Input: part model. Units: mm. Frame: model coordinates. A direction names the side the tool comes from. Round coordinates to 2 decimals unless told otherwise and drop trailing zeros. Loops run counter-clockwise (first coordinate to the right, second up) from the corner with the lowest first, then second, coordinate; pieces in that order, holes last. Notation, with made-up numbers: M 72,83 L 125,83 A9 ccw 125,94 Z; hole C -31.75,66.5 d9. An arc over 180 degrees is marked long. Put each result on its own line as item: value. Start each with the question number.
1) Line query: probe 1 along Y at (x, z) = (-13, 6.5); probe 2 along X at (y, z) = (33, 0.5); probe 3 along Z at (x, y) = (-10, 50). Output: solid intervals per line, ascending.
2) Section D-D on z = 0. Output: boundary loops of the cut face in (x, y).
3) Section A-A on x = 0. Output: boundary loops of the cut face in (y, z).
4) Pin query (flat end, axial travel): pin 1 (10 mm diameter, centred on x = -13, z = 4.5, fed in from -Y); pin 2 (1.5 mm diameter, centred on y = 51.5, z = -1, fed in from +X); pin 3 (5 mm diameter, centred on y = 57, z = 5.5, fed in from -X); pin 4 (12 mm diameter, centred on y = 57, z = -1.5, fed in from -X). Return the tip coordinate at first contact, or that it passes through.
5) Reachability of faces 1 (the face through (0, 77, 5.082)), 2 (the face through (0, 0, 0)) from +Z, -Z, +X, -X, +Y, -Y: full face, straight path, thin tool, end or side. Return the list, or none.
6) Section C-C on y = 16. Output: boundary loops of the cut face in (x, z), plus the area to 3 significant figures.
7) Section B-B on z = 9. Output: boundary loops of the cut face in (x, y), plus the area to 3 significant figures.
from build123d import *

# Parameters (mm, degrees)
SKETCH1_R           = 19.05
BOSS_EXTRUDE1_DEPTH = 76.2
BOSS_EXTRUDE3_DEPTH = 2.54


with BuildPart() as part:
    # Sketch1 → Boss-Extrude1 (new body)
    with BuildSketch(Plane(origin=(0, 0, 0), x_dir=(1, 0, 0), z_dir=(0, 1, 0))):
        with Locations(Location((0, 0, 0), (0, 0, 90))):
            Circle(SKETCH1_R)
    extrude(amount=BOSS_EXTRUDE1_DEPTH)

    # Sketch2 → Boss-Extrude3 (add)
    with BuildSketch(Plane(origin=(0, 76.2, 0), x_dir=(1, 0, 0), z_dir=(0, 1, 0))):
        with BuildLine():
            Line((2.273328114, -5.081659317), (0, -5.081659317))
            Line((0, -5.081659317), (-2.273328114, -5.081659317))
            ThreePointArc((-2.273328114, -5.081659317), (-1.086554166, -9.959754211), (3.048, -7.112))
            ThreePointArc((3.048, -7.112), (2.847754211, -6.025445834), (2.273328114, -5.081659317))
        make_face()
    extrude(amount=BOSS_EXTRUDE3_DEPTH)


solid = part.part
Geometry results:
1. probe 1: y = 0 to 76.2
1. probe 2: x = -19.04 to 19.04
1. probe 3: z = -16.21 to 16.21
2. outline: M -19.05,0 L 19.05,0 L 19.05,76.2 L -19.05,76.2 Z
3. outline: M 0,-19.05 L 76.2,-19.05 L 76.2,5.08 L 78.74,5.08 L 78.74,10.16 L 76.2,10.16 L 76.2,19.05 L 0,19.05 Z
4. pin 1: stops at y = 0
4. pin 2: stops at x = 19.05
4. pin 3: stops at x = -18.81
4. pin 4: stops at x = -19.05
5. face 1: -Z, +X, -X, +Y
5. face 2: +Z, -Z, +X, -X, -Y
6. outline: C 0,0 d38.1
6. area: 1,140 mm²
7. outline: M -16.79,0 L 16.79,0 L 16.79,76.2 L 2.39,76.2 L 2.39,78.74 L -2.39,78.74 L -2.39,76.2 L -16.79,76.2 Z
7. area: 2,570 mm²
